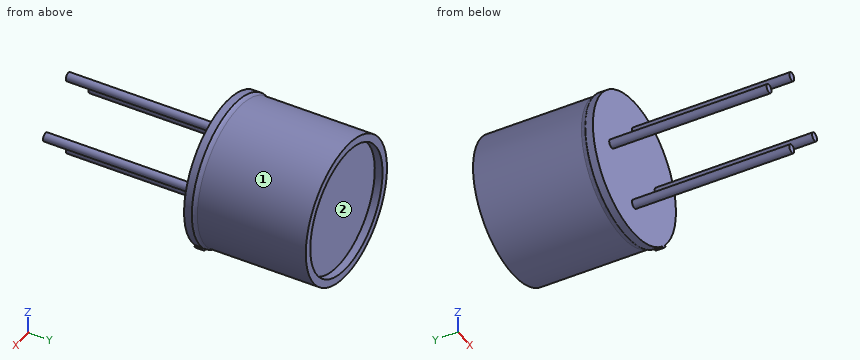
from build123d import *

# Parameters (mm, degrees)
SKETCH1_R           = 4.55
BOSS_EXTRUDE1_DEPTH = 7.8
SKETCH2_R           = 4.050000028
CUT_EXTRUDE1_DEPTH  = 0.5
SKETCH3_R           = 0.275
BOSS_EXTRUDE2_DEPTH = 10.16
SKETCH4_R           = 4.65
BOSS_EXTRUDE3_DEPTH = 0.5
FILLET1_SIZE        = 0.1
FILLET1_SIZE_2      = 0.3
BOSS_EXTRUDE4_DEPTH = 0.5


with BuildPart() as part:
    # Sketch1 → Boss-Extrude1 (new body)
    with BuildSketch(Plane(origin=(0, 0, 0), x_dir=(1, 0, 0), z_dir=(0, 1, 0))):
        with Locations(Location((0, 0, 0), (0, 0, 270))):
            Circle(SKETCH1_R)
    extrude(amount=BOSS_EXTRUDE1_DEPTH)

    # Sketch2 → Cut-Extrude1 (cut)
    with BuildSketch(Plane(origin=(0, 7.8, 0), x_dir=(1, 0, 0), z_dir=(0, 1, 0))):
        with Locations(Location((0, 0, 0), (0, 0, 270))):
            Circle(SKETCH2_R)
    extrude(amount=-CUT_EXTRUDE1_DEPTH, mode=Mode.SUBTRACT)

    # Sketch3 → Boss-Extrude2 (add)
    with BuildSketch(Plane(origin=(0, 0, 0), x_dir=(-1, 0, 0), z_dir=(0, -1, 0))):
        with Locations(Location((0, 2.55, 0), (0, 0, 270))):
            Circle(SKETCH3_R)
        with Locations(Location((2.55, 0, 0), (0, 0, 270))):
            Circle(SKETCH3_R)
        with Locations(Location((0, -2.55, 0), (0, 0, 270))):
            Circle(SKETCH3_R)
        with Locations(Location((-2.55, 0, 0), (0, 0, 270))):
            Circle(SKETCH3_R)
    extrude(amount=BOSS_EXTRUDE2_DEPTH)

    # Sketch4 → Boss-Extrude3 (add)
    with BuildSketch(Plane(origin=(0, 0, 0), x_dir=(-1, 0, 0), z_dir=(0, -1, 0))):
        with Locations(Location((0, 0, 0), (0, 0, 90))):
            Circle(SKETCH4_R)
    extrude(amount=-BOSS_EXTRUDE3_DEPTH)

    # Fillet1
    # an asymmetric fillet: 0.3, 0.1 mm, written as the material it adds along each edge
    with BuildSketch(Plane(origin=(0, 0.5, 0), x_dir=(0, 0, 1), z_dir=(1, 0, 0))) as fillet1_piece_1_section:
        with BuildLine():
            Bezier((4.55 + FILLET1_SIZE, 0), (4.55, 0), (4.55, -FILLET1_SIZE_2), weights=[1, 0.707106781, 1])
            Line((4.55, -FILLET1_SIZE_2), (4.55, 0))
            Line((4.55, 0), (4.55 + FILLET1_SIZE, 0))
        make_face()
    fillet1_piece_1 = revolve(axis=Axis((0, 0.5, 0), (0, -1, 0)), mode=Mode.PRIVATE)
    fillet1_piece_1 = fillet1_piece_1 & Plane(origin=(0, 0.585863309, 0), x_dir=(0, 0, -1), z_dir=(0, -1, 0)) * Cylinder(4.65, 19, mode=Mode.PRIVATE)
    add(fillet1_piece_1)

    # Sketch5 → Boss-Extrude4 (add)
    with BuildSketch(Plane(origin=(0, 0, 0), x_dir=(-1, 0, 0), z_dir=(0, -1, 0))):
        Polygon((-3.075914781, 3.358756928), (-3.217336137, 3.500178284), (-3.500178284, 3.217336137), (-3.358756928, 3.075914781), align=None)
    extrude(amount=-BOSS_EXTRUDE4_DEPTH)


solid = part.part
Check sheet for the modelled part. Datum: model origin and axes. Units: mm. Face numbers are marked on the shaded views. Give positions to 0.01 mm unless a question says otherwise; leave off trailing zeros. Write each loop counter-clockwise with the first axis right and the second up, starting at its lowest first coordinate (ties: lowest second). Pieces come first, ordered by that corner, then holes. Notation, with made-up numbers: (-28, 26.25) -> (-17, 26.25) arc R9 ccw to (-17, 36.25) -> close; hole circle Ø2 at (-34.75, 87). An arc over 180 degrees is marked (long way). Write item = value, one per line.
Item 1: Release check for a two-part mould opening along X. For the marked faces 1 and 2 record: +X half, -X half, draft (parallel to the pull), parting line (faces both ways), or undercut.
Output:
face_1 = parting line
face_2 = undercut
Item 2: Sectioned sample at A-A on y = -2.5. Record the boundary of the cut face in (x, z) (3 decimals).
Output:
outline = circle Ø0.55 at (-2.55, 0); circle Ø0.55 at (0, -2.55); circle Ø0.55 at (0, 2.55); circle Ø0.55 at (2.55, 0)
Item 3: Scan lines: probe 1 along X at (y, z) = (7.7, 0); probe 2 along Y at (x, z) = (-2.5, 0); probe 3 along Y at (x, z) = (-3.75, 2.5). Record each from-to range of solid material in increasing order. Write a range as from..to.
Output:
probe_1 = -4.55..-4.05, 4.05..4.55
probe_2 = -10.16..7.3
probe_3 = 0..7.8
Item 4: Gauge pin test, flat ends, axial feed: pin 1 (1.5 mm diameter, centred on x = -1.5, z = -2.5, fed in from +Y); pin 2 (3 mm diameter, centred on y = 0, z = -2.5, fed in from +X); pin 3 (3 mm diameter, centred on y = -2, z = -0.5, fed in from -X) (3 decimals). Record the tip position at first contact, or that the pin passes through.
Output:
pin_1 = 7.3
pin_2 = 4.54
pin_3 = -2.825
